from build123d import *

# Parameters (mm, degrees)
SKETCH2_W           = 46.3108
SKETCH2_H           = 46.3108
SKETCH2_W_2         = 40.7172
SKETCH2_H_2         = 40.7172
BOSS_EXTRUDE1_DEPTH = 5
SKETCH1_R           = 0.95
CUT_EXTRUDE1_DEPTH  = 6


with BuildPart() as part:
    # Sketch2 → Boss-Extrude1 (new body)
    with BuildSketch(Plane(origin=(0, 0, 0), x_dir=(1, 0, 0), z_dir=(0, 1, 0))):
        Rectangle(SKETCH2_W, SKETCH2_H)
        Rectangle(SKETCH2_W_2, SKETCH2_H_2, mode=Mode.SUBTRACT)
    extrude(amount=BOSS_EXTRUDE1_DEPTH)

    # Sketch1 → Cut-Extrude1 (cut, through all)
    with BuildSketch(Plane(origin=(0, 0, 0), x_dir=(1, 0, 0), z_dir=(0, 1, 0))):
        with Locations((-21.5644, 21.5964)):
            Circle(SKETCH1_R)
        with Locations((-19.0244, 21.5964)):
            Circle(SKETCH1_R)
        with Locations((-21.5644, 19.0564)):
            Circle(SKETCH1_R)
        with Locations((-16.4844, 21.5964)):
            Circle(SKETCH1_R)
        with Locations((-13.9444, 21.5964)):
            Circle(SKETCH1_R)
        with Locations((-11.4044, 21.5964)):
            Circle(SKETCH1_R)
        with Locations((-8.8644, 21.5964)):
            Circle(SKETCH1_R)
        with Locations((-6.3244, 21.5964)):
            Circle(SKETCH1_R)
        with Locations((-3.7844, 21.5964)):
            Circle(SKETCH1_R)
        with Locations((-1.2444, 21.5964)):
            Circle(SKETCH1_R)
        with Locations((1.2956, 21.5964)):
            Circle(SKETCH1_R)
        with Locations((3.8356, 21.5964)):
            Circle(SKETCH1_R)
        with Locations((6.3756, 21.5964)):
            Circle(SKETCH1_R)
        with Locations((8.9156, 21.5964)):
            Circle(SKETCH1_R)
        with Locations((11.4556, 21.5964)):
            Circle(SKETCH1_R)
        with Locations((13.9956, 21.5964)):
            Circle(SKETCH1_R)
        with Locations((16.5356, 21.5964)):
            Circle(SKETCH1_R)
        with Locations((19.0756, 21.5964)):
            Circle(SKETCH1_R)
        with Locations((21.6156, 21.5964)):
            Circle(SKETCH1_R)
        with Locations((-21.5644, 16.5164)):
            Circle(SKETCH1_R)
        with Locations((-21.5644, 13.9764)):
            Circle(SKETCH1_R)
        with Locations((-21.5644, 11.4364)):
            Circle(SKETCH1_R)
        with Locations((-21.5644, 8.8964)):
            Circle(SKETCH1_R)
        with Locations((-21.5644, 6.3564)):
            Circle(SKETCH1_R)
        with Locations((-21.5644, 3.8164)):
            Circle(SKETCH1_R)
        with Locations((-21.5644, 1.2764)):
            Circle(SKETCH1_R)
        with Locations((-21.5644, -1.2636)):
            Circle(SKETCH1_R)
        with Locations((-21.5644, -3.8036)):
            Circle(SKETCH1_R)
        with Locations((-21.5644, -6.3436)):
            Circle(SKETCH1_R)
        with Locations((-21.5644, -8.8836)):
            Circle(SKETCH1_R)
        with Locations((-21.5644, -11.4236)):
            Circle(SKETCH1_R)
        with Locations((-21.5644, -13.9636)):
            Circle(SKETCH1_R)
        with Locations((-21.5644, -16.5036)):
            Circle(SKETCH1_R)
        with Locations((-21.5644, -19.0436)):
            Circle(SKETCH1_R)
        with Locations((-21.5644, -21.5836)):
            Circle(SKETCH1_R)
        with Locations((-19.0244, -21.5836)):
            Circle(SKETCH1_R)
        with Locations((-16.4844, -21.5836)):
            Circle(SKETCH1_R)
        with Locations((-13.9444, -21.5836)):
            Circle(SKETCH1_R)
        with Locations((-11.4044, -21.5836)):
            Circle(SKETCH1_R)
        with Locations((-8.8644, -21.5836)):
            Circle(SKETCH1_R)
        with Locations((-6.3244, -21.5836)):
            Circle(SKETCH1_R)
        with Locations((-3.7844, -21.5836)):
            Circle(SKETCH1_R)
        with Locations((-1.2444, -21.5836)):
            Circle(SKETCH1_R)
        with Locations((1.2956, -21.5836)):
            Circle(SKETCH1_R)
        with Locations((3.8356, -21.5836)):
            Circle(SKETCH1_R)
        with Locations((6.3756, -21.5836)):
            Circle(SKETCH1_R)
        with Locations((8.9156, -21.5836)):
            Circle(SKETCH1_R)
        with Locations((11.4556, -21.5836)):
            Circle(SKETCH1_R)
        with Locations((13.9956, -21.5836)):
            Circle(SKETCH1_R)
        with Locations((16.5356, -21.5836)):
            Circle(SKETCH1_R)
        with Locations((19.0756, -21.5836)):
            Circle(SKETCH1_R)
        with Locations((21.6156, -21.5836)):
            Circle(SKETCH1_R)
        with Locations((21.6156, 19.0564)):
            Circle(SKETCH1_R)
        with Locations((21.6156, 16.5164)):
            Circle(SKETCH1_R)
        with Locations((21.6156, 11.4364)):
            Circle(SKETCH1_R)
        with Locations((21.6156, 8.8964)):
            Circle(SKETCH1_R)
        with Locations((21.6156, 6.3564)):
            Circle(SKETCH1_R)
        with Locations((21.6156, 3.8164)):
            Circle(SKETCH1_R)
        with Locations((21.6156, 1.2764)):
            Circle(SKETCH1_R)
        with Locations((21.6156, -1.2636)):
            Circle(SKETCH1_R)
        with Locations((21.6156, -3.8036)):
            Circle(SKETCH1_R)
        with Locations((21.6156, -6.3436)):
            Circle(SKETCH1_R)
        with Locations((21.6156, -8.8836)):
            Circle(SKETCH1_R)
        with Locations((21.6156, -11.4236)):
            Circle(SKETCH1_R)
        with Locations((21.6156, -13.9636)):
            Circle(SKETCH1_R)
        with Locations((21.6156, -16.5036)):
            Circle(SKETCH1_R)
        with Locations((21.6156, -19.0436)):
            Circle(SKETCH1_R)
        with Locations((21.6156, 13.9764)):
            Circle(SKETCH1_R)
    extrude(amount=CUT_EXTRUDE1_DEPTH, mode=Mode.SUBTRACT)


solid = part.part
Source: CAD feature listing. Evaluate the final solid. Frame: model axes, mm. Give positions to 0.01 mm unless a question says otherwise; leave off trailing zeros. Write each loop counter-clockwise with the first axis right and the second up, starting at its lowest first coordinate (ties: lowest second). Pieces come first, ordered by that corner, then holes. Notation, with made-up numbers: (6, 22) -> (42, 22) arc R6 cw to (42, 28) -> close; hole circle Ø9 at (6.5, -28). An arc over 180 degrees is marked (long way). Return JSON: item names as keys, results as strings. Group by question number.
1. Pin query (flat end, axial travel): pin 1 Ø1.1 at (x, z) = (16.54, -21.6) entering from -Y; pin 2 Ø3 at (x, z) = (-19.02, -21.6) entering from +Y. Return the tip coordinate at first contact, or that it passes through.
2. Section B-B, the plane y = 3.45. Count the separate pieces of the cut face and the enclosed holes in it, then the cut area to 3 significant figures.
3. Section A-A, the plane x = 16.5. Output: boundary loops of the cut face in (y, z).
4. Mould query, pull axis Z, two halves, no side actions, for faces 1 (the face through (0, 2, 23.155)), 2 (the face through (-20.7, 2.5, 16.9)), 3 (the face through (0, 0, -21)). Classes: +Z half, -Z half, draft (parallel to the pull), parting line (faces both ways), or undercut.
5. Material intervals for line 1 (Z direction, x = -14, y = 3.85); line 2 (X direction, y = 3.95, z = -17.5), sorted ascending. Write a range as from..to.
Determined:
{
 "1": {"pin 1": "passes through", "pin 2": "stops at y = 5"},
 "2": {"separate pieces": "1", "enclosed holes": "69", "area": "294 mm2"},
 "3": {"outline": "(0, -23.16) -> (5, -23.16) -> (5, -22.55) -> (0, -22.55) -> close; (0, -20.65) -> (5, -20.65) -> (5, -20.36) -> (0, -20.36) -> close; (0, 20.36) -> (5, 20.36) -> (5, 20.63) -> (0, 20.63) -> close; (0, 22.53) -> (5, 22.53) -> (5, 23.16) -> (0, 23.16) -> close"},
 "4": {"face 1": "+Z half", "face 2": "undercut", "face 3": "draft"},
 "5": {"line 1": "z = -23.16..-22.54, -20.65..-20.36, 20.36..20.64, 22.53..23.16", "line 2": "x = -23.16..-20.36, 20.36..23.16"}
}
